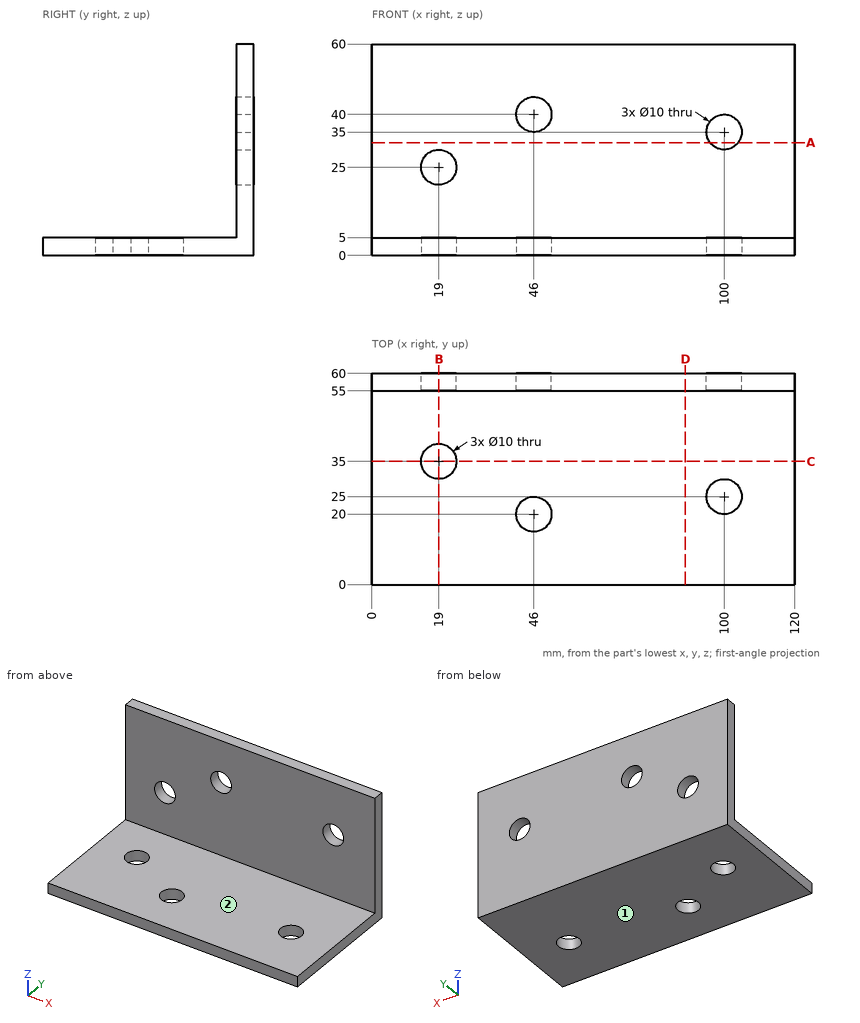
Drawing for the job (mm, zero at the part's lowest x, y, z). A direction names the side the tool comes from. Give positions to 0.01 mm unless a question says otherwise; leave off trailing zeros. Write each loop counter-clockwise with the first axis right and the second up, starting at its lowest first coordinate (ties: lowest second). Pieces come first, ordered by that corner, then holes. Notation, with made-up numbers: M 76.5,56.25 L 113.5,56.25 A22 ccw 113.5,85.25 Z; hole C 63.25,-37.5 d9. An arc over 180 degrees is marked long. Return JSON: item names as keys, results as strings. Group by question number.
(1) 3-axis set-ups, long thin cutter, end or side, ignore diameter. For the marked faces 1 and 2: which of +Z, -Z, +X, -X, +Y, -Y reach the whole face in a straight line?
(2) Band-saw the part on A-A (z = 32). Give the cut face in (x, y), and give its area (3 significant figures).
(3) Drill centre lines: L1, parallel to Z at x = 46, y = 56; L2, parallel to Y at x = 100, z = 3.3; L3, parallel to Z at x = 98, y = 39.5. Where is each one in solid material? Low to high. Write a range as [from, to].
(4) Band-saw the part on B-B (x = 19). Give the cut face in (y, z).
(5) Flat gauge pins, fed straight in: pin 1 Ø2 at (x, z) = (60, 45) entering from -Y; pin 2 Ø13 at (x, y) = (100, 25) entering from +Z. Where does each tip first touch, or does it go through?
(6) Band-saw the part on D-D (x = 89). Give the cut face in (y, z), and give its area (3 significant figures).
(7) Band-saw the part on C-C (y = 35). Give the cut face in (x, z), and give its area (3 significant figures).
Entries:
{
 "1": {"face 1": "-Z, +X, -X, +Y, -Y", "face 2": "+Z, +X, -X, -Y"},
 "2": {"outline": "M 0,55 L 96,55 L 96,60 L 0,60 Z; M 104,55 L 120,55 L 120,60 L 104,60 Z", "area": "560 mm^2"},
 "3": {"L1": "z = [0, 35], [45, 60]", "L2": "y = [0, 20], [30, 60]", "L3": "z = [0, 5]"},
 "4": {"outline": "M 0,0 L 30,0 L 30,5 L 0,5 Z; M 40,0 L 60,0 L 60,20 L 55,20 L 55,5 L 40,5 Z; M 55,30 L 60,30 L 60,60 L 55,60 Z"},
 "5": {"pin 1": "stops at y = 55", "pin 2": "stops at z = 5"},
 "6": {"outline": "M 0,0 L 60,0 L 60,60 L 55,60 L 55,5 L 0,5 Z", "area": "575 mm^2"},
 "7": {"outline": "M 0,0 L 14,0 L 14,5 L 0,5 Z; M 24,0 L 120,0 L 120,5 L 24,5 Z", "area": "550 mm^2"}
}
